Autodesk Inventor part; units mm, degrees
ref_plane "YZ Plane" through (0, 0, 0) normal (1, 0, 0) x (0, 1, 0)
ref_plane "XZ Plane" through (0, 0, 0) normal (0, 1, 0) x (-1, 0, 0)
ref_plane "XY Plane" through (0, 0, 0) normal (0, 0, 1) x (1, 0, 0)
sketch "Sketch1" plane through (0, 0, 0) normal (0, 1, 0) x (-1, 0, 0)
  line L0 (-42.5, -40) -> (42.5, -40)
  line L1 (42.5, -40) -> (42.5, 40)
  line L2 (42.5, 40) -> (-42.5, 40)
  line L3 (-42.5, 40) -> (-42.5, -40)
  line L4 (-42.5, -40) -> (42.5, 40) construction
  line L5 (42.5, -40) -> (-42.5, 40) construction
  circle A0 centre (0, 0) radius 14
  dimension "d0" = 85
  dimension "d1" = 80
  dimension "d4" = 28
extrude "Extrusion1" add sketch "Sketch1" along normal blind 6
properties part number "segment0b" material "Plywood, Finish"
Work out the finished part from the listing and answer in its coordinate system (mm). Give positions to 0.01 mm unless a question says otherwise; leave off trailing zeros. Write each loop counter-clockwise with the first axis right and the second up, starting at its lowest first coordinate (ties: lowest second). Pieces come first, ordered by that corner, then holes.
Q1. Straight lines are drawn through the part: L1, parallel to Z at x = 0, y = 1.2; L2, parallel to Z at x = 5, y = 4.75; L3, parallel to X at y = 3.95, z = 6. For each, find the intervals that lie inside material, in ascending order.
Answer:
L1: z = -40 to -14, 14 to 40
L2: z = -40 to -13.08, 13.08 to 40
L3: x = -42.5 to -12.65, 12.65 to 42.5
Q2. The part is cut by section A-A on z = 0. Give the vertices of the cut face in (x, y), and give its area (3 significant figures).
Answer:
outline: (-42.5, 0) - (-14, 0) - (-14, 6) - (-42.5, 6) - close; (14, 0) - (42.5, 0) - (42.5, 6) - (14, 6) - close
area: 342 mm2
Q3. The part is cut by section C-C on y = 2.35. Give the vertices of the cut face in (x, z), and give its area (3 significant figures).
Answer:
outline: (-42.5, -40) - (42.5, -40) - (42.5, 40) - (-42.5, 40) - close; hole circle Ø28 at (0, 0)
area: 6,180 mm2
Q4. For a pull along X with two mould halves and no side action, classify faces 1 (the face through (-1, 3, 40)), 2 (the face through (-42.5, 3, -1)), 3 (the face through (-12.932, 2.958, 5.362)) as released by +X, released by -X, zero draft, split by the parting line, or undercut.
Answer:
face 1: zero draft
face 2: released by -X
face 3: undercut
Q5. The part is cut by section B-B on x = 0. Give the vertices of the cut face in (y, z).
Answer:
outline: (0, -40) - (6, -40) - (6, -14) - (0, -14) - close; (0, 14) - (6, 14) - (6, 40) - (0, 40) - close
